Autodesk Inventor part; units mm, degrees
ref_plane "Start Plane" through (0, 0, -1.1225) normal (0, 0, 1) x (1, 0, 0)
ref_plane "End Plane" through (0, 0, 10) normal (0, 0, 1) x (1, 0, 0)
ref_plane "Work Plane4" through (0, 1.5875, -1.5875) normal (0, -0.7071, -0.7071) x (1, 0, 0)
ref_plane "Start Plane" through (0, 0, -1.1225) normal (0, 0, 1) x (1, 0, 0)
ref_plane "End Plane" through (0, 0, 10) normal (0, 0, 1) x (1, 0, 0)
sketch "Sketch" plane through (0, 0, 0) normal (0, 0, 1) x (1, 0, 0)
  circle A0 centre (0, 0) radius 1.5875
  dimension "d0" = 3.175
extrude "Body" add sketch "Sketch" along normal up to surface (11.1225 mm away) from surface at -1.1225
sketch "Sketch2" plane through (0, 0, 0) normal (0, 0, 1) x (1, 0, 0)
  line L0 (0, 0) -> (10, 0)
ref_plane "Work Plane3" through (0, 0, 0) normal (0, -1, 0) x (1, 0, 0)
sketch "Sketch3" plane through (0, 0, 0) normal (0, -1, 0) x (1, 0, 0)
  line L0 (-2, -1.1225) -> (12, -1.1225)
  line L1 (-2, 10) -> (12, 10)
  dimension "d7" = 11.1225
ref_plane "Work Plane4" through (0, 1.5875, -1.5875) normal (0, -0.7071, -0.7071) x (1, 0, 0)
split "Split1" plane through (0, 1.5875, -1.5875) removes the side toward (0, -0.7071, -0.7071)
ref_plane "Work Plane5" through (1.5875, 0, -1.5875) normal (-0.7071, 0, -0.7071) x (-0.7071, 0, 0.7071)
split "Split2" plane through (1.5875, 0, -1.5875) removes the side toward (-0.7071, 0, -0.7071)
equation "\"d0\" = Diam"
equation "\"d1\" = G_L"
equation "\"Diam\" = 3.175"
equation "\"G_L\" = d7"
equation "\"G_OFFSET_START\" = 1.12253"
equation "\"G_OFFSET_END\" = 0"
equation "\"d4\" = -G_OFFSET_START"
equation "\"d5\" = G_OFFSET_END + B_L"
equation "\"B_L\" = 10"
properties part number "ANSI/AISC Rolled Steel - 1/8-0,438, RB" material "Steel, Mild"
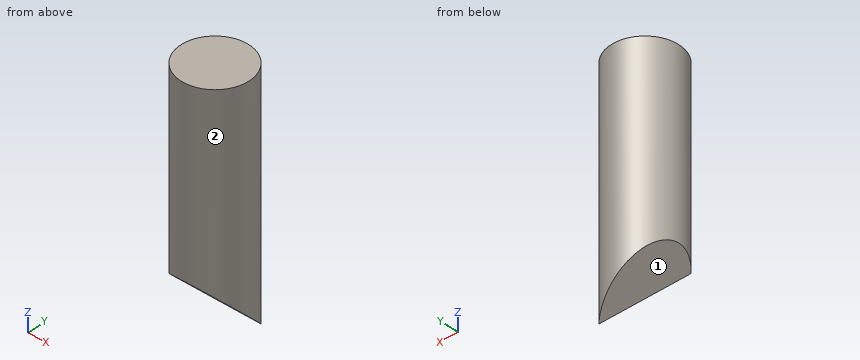
Read the model definition and answer for the solid it produces. Units are mm, in the model's axes. Face numbers are marked on the shaded views. Round coordinates to 2 decimals unless told otherwise and drop trailing zeros. Order: outer loops, then holes, each group sorted by start corner. A loop starts at its lowest first (then second) coordinate and runs counter-clockwise, first axis right, second up. Notation, with made-up numbers: (0.5, 39.25) - (36.5, 39.25) arc R19 cw to (36.5, 75.25) - close; hole circle Ø4 at (34.25, 21). An arc over 180 degrees is marked (long way). Use one line per item in the form item = value. Start each with the question number.
(1) Find the intervals of material crossed by line 1 along Z through (x, y) = (0.15, -0.55); line 2 along Y through (x, z) = (0.7, 8.5); line 3 along Z through (x, y) = (-1.05, 0.75), in increasing order. Write a range as from..to.
(2) Flat-ended cylindrical pins translate along their axes: pin 1 Ø1.5 at (x, z) = (1, 2.5) entering from -Y; pin 2 Ø1 at (y, z) = (1, 1.5) entering from -X. Find the tip coordinate at first contact, or state that the pin passes through.
(3) Determine the mould class of the marked faces 1 and 2 for opening direction Y: +Y half, -Y half, draft (parallel to the pull), parting line (faces both ways), or undercut.
(4) The part is cut by section A-A (x = 0). Give the vertices of the cut face in (y, z), then the cut area to 3 significant figures.
(5) The part is cut by section C-C (z = 5). Give the vertices of the cut face in (x, y) (1 decimal), then the cut area to 3 significant figures.
Checked values:
q1.line_1 = 0.55..10
q1.line_2 = -1.42..1.42
q1.line_3 = 1.05..10
q2.pin_1 = -1.57
q2.pin_2 = -1.51
q3.face_1 = draft
q3.face_2 = parting line
q4.outline = (-1.59, 1.59) - (0, 0) - (1.59, 0) - (1.59, 10) - (-1.59, 10) - close
q4.area = 30.5 mm^2
q5.outline = circle Ø3.2 at (0, 0)
q5.area = 7.92 mm^2
